Read the model definition and answer for the solid it produces. Units are mm, in the model's axes. A direction names the side the tool comes from. Coordinates: 2 decimals unless noted, no trailing zeros. Write each loop counter-clockwise with the first axis right and the second up, starting at its lowest first coordinate (ties: lowest second). Pieces come first, ordered by that corner, then holes. Notation, with made-up numbers: (-9, -11.75) - (30, -11.75) arc R23 cw to (30, 11.25) - close; hole circle Ø7 at (65.5, 72). An arc over 180 degrees is marked (long way). Return JSON: item names as keys, results as strings.
```python
from build123d import *

# Parameters (mm, degrees)
EXTRUDE_1_DEPTH     = 10
SKETCH_2_W          = 2.859550618
SKETCH_2_H          = 5.796062829
EXTRUDE_2_DEPTH     = 10
SKETCH_11_W         = 2.859550618
SKETCH_11_H         = 5.796062829
CUT_EXTRUDE_8_DEPTH = 2
SKETCH_12_W         = 2.859550618
SKETCH_12_H         = 5.796062829
CUT_EXTRUDE_9_DEPTH = 2


with BuildPart() as part:
    # 草圖1 → 填料-伸長1 (new body)
    with BuildSketch(Plane.XY):
        with BuildLine():
            Line((0, 0), (-8.942496936, 0))
            Line((-8.942496936, 0), (-8.942496936, -5.796062829))
            Line((-8.942496936, -5.796062829), (0, -5.796062829))
            ThreePointArc((0, -5.796062829), (-11.918722494, -13.716380039), (-26.209286831, -14.469468031))
            Line((-26.209286831, -14.469468031), (-24.418965375, -11.038018573))
            ThreePointArc((-24.418965375, -11.038018573), (-21.767209123, -1.713427654), (-24.418965375, 7.611163265))
            Line((-24.418965375, 7.611163265), (-26.209286831, 11.266402905))
            ThreePointArc((-26.209286831, 11.266402905), (-11.360125695, 9.691512317), (0, 0))
        make_face()
    extrude(amount=EXTRUDE_1_DEPTH)

    # 草圖2 → 填料-伸長2 (add)
    with BuildSketch(Plane.XY):
        with Locations((-1.429775309, -2.898031415)):
            Rectangle(SKETCH_2_W, SKETCH_2_H)
    extrude(amount=EXTRUDE_2_DEPTH)

    # 草圖11 → 除料-伸長8 (cut)
    with BuildSketch(Plane.XY.offset(10)):
        with Locations((-1.429775309, -2.898031415)):
            Rectangle(SKETCH_11_W, SKETCH_11_H)
    extrude(amount=-CUT_EXTRUDE_8_DEPTH, mode=Mode.SUBTRACT)

    # 草圖12 → 除料-伸長9 (cut)
    with BuildSketch(Plane(origin=(0, 0, 0), x_dir=(-1, 0, 0), z_dir=(0, 0, -1))):
        with Locations((1.429775309, -2.898031415)):
            Rectangle(SKETCH_12_W, SKETCH_12_H)
    extrude(amount=-CUT_EXTRUDE_9_DEPTH, mode=Mode.SUBTRACT)


solid = part.part
```
(1) Determine the mould class of faces 5 (the face through (-13, -1, 0)), 6 (the face through (-11.555, 9.775, 4.93)), 7 (the face through (-8.942, -3, 5)) for opening direction Y: +Y half, -Y half, draft (parallel to the pull), parting line (faces both ways), or undercut.
Answer:
{"face 5": "draft", "face 6": "+Y half", "face 7": "undercut"}
(2) Flat-ended cylindrical pins translate along their axes: P1, Ø0.9, axis at x = -2, y = -2, coming from the +Z side; P2, Ø3, axis at x = -2, y = -3.5, coming from the -Z side; P3, Ø6, axis at y = 2.5, z = 6.5, coming from the -X side. Find the tip coordinate at first contact, or state that the pin passes through.
Answer:
{"P1": "z = 8", "P2": "z = 2", "P3": "x = -23.3"}
(3) A cutting plane is placed at B-B (x = -4.75). Determine the outline of the cut face in (y, z), and give its area (3 significant figures).
Answer:
{"outline": "(-10.09, 0) - (-5.8, 0) - (-5.8, 10) - (-10.09, 10) - close; (0, 0) - (5.54, 0) - (5.54, 10) - (0, 10) - close", "area": "98.3 mm²"}
(4) A cutting plane is placed at C-C (y = -1.25). Determine the outline of the cut face in (x, z), and give its area (3 significant figures).
Answer:
{"outline": "(-21.77, 0) - (-8.94, 0) - (-8.94, 10) - (-21.77, 10) - close; (-2.86, 2) - (0, 2) - (0, 8) - (-2.86, 8) - close", "area": "145 mm²"}
(5) Which of the six approach directions +Z, -Z, +X, -X, +Y, -Y give full straight-line access (tool end or side, diameter ignored) to faces 1 (the face through (-1, -3, 2)), 2 (the face through (-25.3, 9.41, 4.93)), 3 (the face through (-1, -3, 8)), 4 (the face through (-2.86, -3, 5))?
Answer:
{"face 1": "-Z, +X", "face 2": "+Z, -Z, -X", "face 3": "+Z, +X", "face 4": "+Z, -Z"}
(6) A cutting plane is placed at D-D (z = 8.75). Determine the outline of the cut face in (x, y), and give its area (3 significant figures).
Answer:
{"outline": "(-26.21, -14.47) arc R27.13 ccw to (0, -5.8) - (-8.94, -5.8) - (-8.94, 0) - (0, 0) arc R25.24 ccw to (-26.21, 11.27) - (-24.42, 7.61) arc R17.72 cw to (-24.42, -11.04) - close", "area": "444 mm²"}
(7) Straight lines are drawn through the part: line 1 (Y direction, x = -24, z = 3.75); line 2 (Y direction, x = -5.25, z = 4.25); line 3 (X direction, y = 1.25, z = 4). For each, find the intervals that lie inside material, in ascending order. Write a range as from..to.
Answer:
{"line 1": "-14.86..-10.32, 6.9..11.6", "line 2": "-10.44..-5.8, 0..5.96", "line 3": "-22.02..-0.84"}
(8) A cutting plane is placed at A-A (z = 4). Determine the outline of the cut face in (x, y).
Answer:
{"outline": "(-26.21, -14.47) arc R27.13 ccw to (0, -5.8) - (0, 0) arc R25.24 ccw to (-26.21, 11.27) - (-24.42, 7.61) arc R17.72 cw to (-24.42, -11.04) - close; hole (-8.94, -5.8) - (-2.86, -5.8) - (-2.86, 0) - (-8.94, 0) - close"}
